from build123d import *

# Parameters (mm, degrees)
F2_W     = 127.7
F2_H     = 85
F2_R     = 17.85
F3_DEPTH = 2


# Not quite as in the source:
# - a feature names something its author has since deleted; it is built from what else it names


with BuildPart() as f3:
    # F2 (on offset) → F3 (new body)
    with BuildSketch(Plane.XY.offset(2)):
        Rectangle(F2_W, F2_H)
        Circle(F2_R, mode=Mode.SUBTRACT)
    extrude(amount=-F3_DEPTH)


solid = f3.part
Geometry: final body of the model. Coordinates: model frame, mm. Coordinates: 2 decimals unless noted, no trailing zeros. Order: outer loops, then holes, each group sorted by start corner. A loop starts at its lowest first (then second) coordinate and runs counter-clockwise, first axis right, second up.
1) Section C-C (z = 1.25). Return loops of the section in (x, y).
Result sheet:
outline: (-63.85, -42.5) - (63.85, -42.5) - (63.85, 42.5) - (-63.85, 42.5) - close; hole circle Ø35.7 at (0, 0)
2) Draft query along X for faces 1 (the cylindrical face through (-17.833, 0.785, 1.014)), 2 (the flat face through (-15, 10, 2)). Return one class per face: released by +X, released by -X, zero draft, split by the parting line, or undercut.
Result sheet:
face 1: undercut
face 2: zero draft
3) Section A-A (y = 0). Return loops of the section in (x, z).
Result sheet:
outline: (-63.85, 0) - (-17.85, 0) - (-17.85, 2) - (-63.85, 2) - close; (17.85, 0) - (63.85, 0) - (63.85, 2) - (17.85, 2) - close
4) Ray query, probe 1 along Y at (x, z) = (0, 0.85); probe 2 along X at (y, z) = (-1.5, 1.6); probe 3 along X at (y, z) = (14, 1). Return the intervals inside material, ascending.
Result sheet:
probe 1: y = -42.5 to -17.85, 17.85 to 42.5
probe 2: x = -63.85 to -17.79, 17.79 to 63.85
probe 3: x = -63.85 to -11.07, 11.07 to 63.85
5) Section B-B (x = 0). Return loops of the section in (y, z), then the cut area to 3 significant figures.
Result sheet:
outline: (-42.5, 0) - (-17.85, 0) - (-17.85, 2) - (-42.5, 2) - close; (17.85, 0) - (42.5, 0) - (42.5, 2) - (17.85, 2) - close
area: 98.6 mm2
